Verification items for the finished model (mm, model axes). A direction names the side the tool comes from. Coordinates: 2 decimals unless noted, no trailing zeros. Order: outer loops, then holes, each group sorted by start corner. A loop starts at its lowest first (then second) coordinate and runs counter-clockwise, first axis right, second up. Notation, with made-up numbers: M 27,8.25 L 84,8.25 A19 cw 84,20.25 Z; hole C 24.5,22.5 d9. An arc over 180 degrees is marked long. Write item = value, one per line.
Autodesk Inventor part; units mm, degrees
ref_plane "Plano de trabajo1" through (0, -7.5, 0) normal (1, 0, 0) x (0, 0, -1)
ref_plane "YZ Plane" through (0, 0, 0) normal (1, 0, 0) x (0, 1, 0)
ref_plane "XZ Plane" through (0, 0, 0) normal (0, 1, 0) x (-1, 0, 0)
sketch "Boceto1" plane through (0, 0, 0) normal (0, 0, 1) x (1, 0, 0)
  line L0 (-7.5, -7.5) -> (7.5, -7.5)
  line L1 (7.5, -7.5) -> (7.5, 7.5)
  line L2 (7.5, 7.5) -> (-7.5, 7.5)
  line L3 (-7.5, 7.5) -> (-7.5, -7.5)
  line L4 (-7.5, -7.5) -> (7.5, 7.5) construction
  line L5 (7.5, -7.5) -> (-7.5, 7.5) construction
  point P0 (0, 0)
  dimension "d0" = 15
extrude "Extrusión1" add sketch "Boceto1" against normal blind 5
ref_plane "Plano de trabajo1" through (0, -7.5, 0) normal (1, 0, 0) x (0, 0, -1)
sketch "Boceto2" plane through (0, -7.5, 0) normal (1, 0, 0) x (0, 0, -1)
  line L0 (5, 15) -> (5, 0)
  arc A0 (14, 7.5) -> (5, 16.5) centre (5, 7.5) ccw
  line L1 (5, 7.5) -> (14, 7.5)
  line L2 (5, 7.5) -> (5, 16.5)
  point P0 (0, 7.5)
  dimension "d5" = 9
revolve "Revolución1" add sketch "Boceto2" angle 360 about axis through (0, 0, -5) along (0, 0, -1)
sketch "Boceto3" plane through (0, 0, 0) normal (0, 0, 1) x (1, 0, 0)
  line L0 (-7.5, 7.5) -> (-7.5, -7.5)
  line L1 (-7.5, 7.5) -> (7.5, 7.5)
  line L2 (7.5, 7.5) -> (7.5, -7.5)
  line L3 (7.5, -7.5) -> (-7.5, -7.5)
  line L4 (-7.5, -7.5) -> (-7.5, 7.5)
  circle A0 centre (0, 0) radius 9
  arc A1 (-4.9749, -7.5) -> (4.9749, -7.5) centre (0, 0) ccw
  line L5 (-7.5, -7.5) -> (7.5, -7.5)
  line L6 (7.5, -7.5) -> (7.5, 7.5)
  line L7 (-7.5, 7.5) -> (-4, 7.5)
  line L8 (-4, 7.5) -> (-4, 4)
  line L9 (-4, 4) -> (-7.5, 4)
  line L10 (-7.5, 4) -> (-7.5, 7.5)
  line L11 (-7.5, -7.5) -> (-7.5, -4)
  line L12 (-7.5, -4) -> (-4, -4)
  line L13 (-4, -4) -> (-4, -7.5)
  line L14 (-4, -7.5) -> (-7.5, -7.5)
  line L15 (7.5, -7.5) -> (4, -7.5)
  line L16 (4, -7.5) -> (4, -4)
  line L17 (4, -4) -> (7.5, -4)
  line L18 (7.5, -4) -> (7.5, -7.5)
  line L19 (7.5, 7.5) -> (7.5, 4)
  line L20 (7.5, 4) -> (4, 4)
  line L21 (4, 4) -> (4, 7.5)
  line L22 (4, 7.5) -> (7.5, 7.5)
  point P0 (-7.5, -7.5)
  point P1 (7.5, -4.9749)
  point P2 (7.5, 4.9749)
  point P3 (7.5, -4)
  point P4 (4, -7.5)
  point P5 (4, 7.5)
  point P6 (7.5, 4)
  dimension "d9" = 3.5
  dimension "d12" = 360
extrude "Extrusión2" cut sketch "Boceto3" against normal up to next contours L0 A0 | L0 A0 L1 L8 L9 | L12 L13 L3 A0 L0 | L0 L1 A0 | A0 L3 L0 | A0 L1 | L3 A0 | A0 L2 L20 L21 L1 | L1 L2 A0 | A0 L2 L3 | L3 L16 L17 L2 A0 | A0 L2
sketch "Boceto4" plane through (0, 0, 0) normal (0, 0, 1) x (1, 0, 0)
  line L0 (-7.5, -7.5) -> (7.5, -7.5)
  line L1 (7.5, -7.5) -> (7.5, 7.5)
  line L2 (7.5, 7.5) -> (-7.5, 7.5)
  line L3 (-7.5, 7.5) -> (-7.5, -7.5)
  line L4 (-7.5, -7.5) -> (7.5, 7.5) construction
  line L5 (7.5, -7.5) -> (-7.5, 7.5) construction
  line L6 (4, 7.5) -> (-4, 7.5)
  line L7 (7.5, -4) -> (7.5, 4)
  point P0 (0, 0)
extrude "Extrusión3" add sketch "Boceto4" against normal blind 3
sketch "Boceto5" plane through (0, 0, 0) normal (0, 0, 1) x (1, 0, 0)
  circle A0 centre (-6, -6) radius 0.75
  circle A1 centre (6, -6) radius 0.75
  circle A2 centre (6, 6) radius 0.75
  circle A3 centre (-6, 6) radius 0.75
  circle A4 centre (0, 0) radius 1.6
  dimension "d16" = 1.5
  dimension "d19" = 360
  dimension "d25" = 3.2
extrude "Extrusión4" cut sketch "Boceto5" against normal up to next
sketch "Boceto6" plane through (-7.5, -7.5, 0) normal (0, -1, 0) x (1, 0, 0)
  line L0 (5.9, 7) -> (5.9, -7)
  line L1 (5.9, -7) -> (9.1, -7)
  line L2 (9.1, -7) -> (9.1, 7)
  line L3 (9.1, 7) -> (5.9, 7)
  line L4 (5.9, 7) -> (9.1, -7) construction
  line L5 (5.9, -7) -> (9.1, 7) construction
  point P0 (7.5, 0)
  point P1 (7.5, 0)
  dimension "d26" = 3.2
  dimension "d27" = 7
extrude "Extrusión5" cut sketch "Boceto6" against normal blind 7.5
properties part number "sujecion_cable_2"
Item 1: Sectioned sample at D-D, the plane y = -6. Enter the section's corners in (x, z), then the cut area to 3 significant figures.
Report:
outline = M -7.5,-3 L -6.75,-3 L -6.75,0 L -7.5,0 Z; M -5.25,-3 L -4,-3 L -4,-10.39 A6.71 ccw 4,-10.39 L 4,-3 L 5.25,-3 L 5.25,0 L 1.6,0 L 1.6,-7 L -1.6,-7 L -1.6,0 L -5.25,0 Z; M 6.75,-3 L 7.5,-3 L 7.5,0 L 6.75,0 Z
area = 79.9 mm^2
Item 2: Scan lines: L1, parallel to Y at x = -6, z = -1.65; L2, parallel to Y at x = 0, z = -9.5. Record each from-to range of solid material in increasing order. Write a range as from..to.
Report:
L1 = -7.5..-6.75, -5.25..5.25, 6.75..7.5
L2 = -7.5..-1.6, 1.6..7.5
Item 3: Sectioned sample at C-C, the plane z = -1.75. Enter the section's corners in (x, y).
Report:
outline = M -7.5,-7.5 L -1.6,-7.5 L -1.6,0 A1.6 cw 1.6,0 L 1.6,-7.5 L 7.5,-7.5 L 7.5,7.5 L -7.5,7.5 Z; hole C -6,-6 d1.5; hole C -6,6 d1.5; hole C 6,-6 d1.5; hole C 6,6 d1.5
Item 4: Tool access check on faces 4 (the flat face through (6, -4, -6)), 5 (the flat face through (-6, -4, -6)), 6 (the cylindrical face through (-6.75, 6.03, -1.48)), 7 (the flat face through (0, -5, -7)), 8 (the flat face through (-5, 5, -3)). Record the directions out of +Z, -Z, +X, -X, +Y, -Y that give a thin tool (end or side, any length) a straight path to the whole face; none if there is none.
Report:
face_4 = -Z, +X, -Y
face_5 = -Z, -X, -Y
face_6 = +Z, -Z
face_7 = +Z, -Y
face_8 = -Z, -X, +Y
Item 5: Gauge pin test, flat ends, axial feed: pin 1 (0.9 mm diameter, centred on x = -6, y = -6, fed in from +Z); pin 2 (3 mm diameter, centred on y = -6, z = -7.5, fed in from -X); pin 3 (3 mm diameter, centred on y = 5, z = -7, fed in from +X); pin 4 (3 mm diameter, centred on x = -6.5, y = 5, fed in from -Z). Record the tip position at first contact, or that the pin passes through.
Report:
pin_1 = through
pin_2 = -4
pin_3 = 7.5
pin_4 = -11
Item 6: Sectioned sample at A-A, the plane z = -7.25. Enter the section's corners in (x, y).
Report:
outline = M -7.5,-4 L -4,-4 L -4,-7.5 L 4,-7.5 L 4,-4 L 7.5,-4 L 7.5,4 L 4,4 L 4,7.5 L -4,7.5 L -4,4 L -7.5,4 Z; hole C 0,0 d3.2
Item 7: Sectioned sample at B-B, the plane x = 0. Enter the section's corners in (y, z).
Report:
outline = M -7.5,-9.97 A9 ccw -1.6,-13.86 L -1.6,-7 L -7.5,-7 Z; M 1.6,-13.86 A9 ccw 7.5,-9.97 L 7.5,0 L 1.6,0 Z
Item 8: Release check for a two-part mould opening along X. For faces 1 (the flat face through (4, 6, -6)), 2 (the flat face through (6, 4, -6)), 3 (the flat face through (1.6, -4, -4)) record: pulls with the +X half, pulls with the -X half, needs draft (parallel to the pull), parting line crosses it, or undercut.
Report:
face_1 = pulls with the +X half
face_2 = needs draft
face_3 = undercut
